Part model, mm, in its own coordinate system. Coordinates: 2 decimals unless noted, no trailing zeros. Order: outer loops, then holes, each group sorted by start corner. A loop starts at its lowest first (then second) coordinate and runs counter-clockwise, first axis right, second up.
from build123d import *

# Parameters (mm, degrees)
BOSS_EXTRUDE1_DEPTH = 0.254
SKETCH2_R           = 4.699
CUT_EXTRUDE1_DEPTH  = 1.254
SKETCH3_W           = 2.54
SKETCH3_H           = 0.635
CUT_EXTRUDE2_DEPTH  = 1.254
CUT_EXTRUDE4_DEPTH  = 1.254
CUT_EXTRUDE5_DEPTH  = 1.254


with BuildPart() as part:
    # Sketch1 → Boss-Extrude1 (new body)
    with BuildSketch(Plane.XY):
        with BuildLine():
            Line((67.21146711, 76.191723231), (8.696654013, 17.676910134))
            Line((8.696654013, 17.676910134), (7.228954972, 14.133571205))
            ThreePointArc((7.228954972, 14.133571205), (14.666587579, 6.075099489), (15.105587123, -4.88230096))
            Line((15.105587123, -4.88230096), (18.648926052, -6.35))
            Line((18.648926052, -6.35), (101.401368334, -6.35))
            ThreePointArc((101.401368334, -6.35), (93.866160503, 38.880636728), (67.21146711, 76.191723231))
        make_face()
        with BuildLine():
            Line((88.672924278, 6.35), (27.86051193, 6.35))
            ThreePointArc((27.86051193, 6.35), (26.399857642, 10.93517908), (24.190484974, 15.210228852))
            Line((24.190484974, 15.210228852), (67.191354125, 58.211098004))
            ThreePointArc((67.191354125, 58.211098004), (82.13289044, 34.020557137), (88.672924278, 6.35))
        make_face(mode=Mode.SUBTRACT)
    extrude(amount=BOSS_EXTRUDE1_DEPTH)

    # Sketch2 → Cut-Extrude1 (cut, through all)
    with BuildSketch(Plane.XY.offset(0.254)):
        with Locations((22.225, 0)):
            Circle(SKETCH2_R)
        with Locations((36.195, 0)):
            Circle(SKETCH2_R)
        with Locations((61.722, 0)):
            Circle(SKETCH2_R)
        with Locations((75.692, 0)):
            Circle(SKETCH2_R)
        with Locations((95.25, 0)):
            Circle(SKETCH2_R)
        with Locations((15.715448212, 15.715448212)):
            Circle(SKETCH2_R)
        with Locations((25.593729945, 25.593729945)):
            Circle(SKETCH2_R)
        with Locations((43.644044748, 43.644044748)):
            Circle(SKETCH2_R)
        with Locations((53.522326482, 53.522326482)):
            Circle(SKETCH2_R)
        with Locations((92.004434954, 24.652514046)):
            Circle(SKETCH2_R)
        with Locations((82.48891971, 47.625)):
            Circle(SKETCH2_R)
        with Locations((67.351920908, 67.351920908)):
            Circle(SKETCH2_R)
    extrude(amount=-CUT_EXTRUDE1_DEPTH, mode=Mode.SUBTRACT)

    # Sketch3 → Cut-Extrude2 (cut, through all)
    with BuildSketch(Plane.XY.offset(0.254)):
        Polygon((15.266435406, 24.246691527), (17.06248663, 26.042742751), (17.511499436, 25.593729945), (15.715448212, 23.797678721), align=None)
        Polygon((44.991083167, 53.971339288), (43.195031942, 52.175288063), (43.644044748, 51.726275257), (45.440095973, 53.522326482), align=None)
        with Locations((29.21, -6.0325)):
            Rectangle(SKETCH3_W, SKETCH3_H)
        with Locations((68.707, -6.0325)):
            Rectangle(SKETCH3_W, SKETCH3_H)
        Polygon((29.230733674, 38.210989795), (31.026784898, 40.007041019), (31.475797704, 39.558028213), (29.67974648, 37.761976989), align=None)
        Polygon((56.845021246, 65.825277367), (55.048970022, 64.029226143), (55.497982828, 63.580213337), (57.294034052, 65.376264561), align=None)
        with Locations((48.9585, -6.0325)):
            Rectangle(SKETCH3_W, SKETCH3_H)
        with Locations((85.471, -6.0325)):
            Rectangle(SKETCH3_W, SKETCH3_H)
        Polygon((99.935462164, 14.437711971), (100.266998693, 11.919442024), (101.526133667, 12.085210288), (101.194597138, 14.603480236), align=None)
        Polygon((93.765504959, 37.464305742), (94.938831965, 37.950313702), (93.966816047, 40.296967714), (92.793489041, 39.810959755), align=None)
        Polygon((79.327792988, 62.471156422), (80.874047017, 60.456038938), (81.88160576, 61.229165953), (80.33535173, 63.244283437), align=None)
        Polygon((13.593916116, 7.005422516), (14.565932035, 4.658768503), (15.739259041, 5.144776462), (14.767243123, 7.491430475), align=None)
    extrude(amount=-CUT_EXTRUDE2_DEPTH, mode=Mode.SUBTRACT)

    # Sketch6 → Cut-Extrude4 (cut, through all)
    with BuildSketch(Plane.XY.offset(0.254)):
        with BuildLine():
            Line((22.27103518, 28.91642471), (40.321349984, 46.966739513))
            ThreePointArc((40.321349984, 46.966739513), (46.966739513, 46.966739513), (46.966739513, 40.321349984))
            Line((46.966739513, 40.321349984), (28.91642471, 22.27103518))
            ThreePointArc((28.91642471, 22.27103518), (22.27103518, 22.27103518), (22.27103518, 28.91642471))
        make_face()
        with BuildLine():
            Line((50.199631717, 56.845021246), (64.029226143, 70.674615673))
            ThreePointArc((64.029226143, 70.674615673), (70.674615673, 70.674615673), (70.674615673, 64.029226143))
            Line((70.674615673, 64.029226143), (56.845021246, 50.199631717))
            ThreePointArc((56.845021246, 50.199631717), (50.199631717, 50.199631717), (50.199631717, 56.845021246))
        make_face()
        with BuildLine():
            Line((61.722, -4.699), (36.195, -4.699))
            ThreePointArc((36.195, -4.699), (31.496, 0), (36.195, 4.699))
            Line((36.195, 4.699), (61.722, 4.699))
            ThreePointArc((61.722, 4.699), (66.421, 0), (61.722, -4.699))
        make_face()
        with BuildLine():
            Line((95.25, -4.699), (75.692, -4.699))
            ThreePointArc((75.692, -4.699), (70.993, 0), (75.692, 4.699))
            Line((75.692, 4.699), (95.25, 4.699))
            ThreePointArc((95.25, 4.699), (99.949, 0), (95.25, -4.699))
        make_face()
        with BuildLine():
            ThreePointArc((96.543320412, 25.868704739), (92.340835395, 38.248826381), (86.558373083, 49.9745))
            ThreePointArc((86.558373083, 49.9745), (80.13941971, 51.694453372), (78.419466338, 45.2755))
            ThreePointArc((78.419466338, 45.2755), (83.658215548, 34.652367484), (87.465549496, 23.436323353))
            ThreePointArc((87.465549496, 23.436323353), (93.220625647, 20.113628588), (96.543320412, 25.868704739))
        make_face()
    extrude(amount=-CUT_EXTRUDE4_DEPTH, mode=Mode.SUBTRACT)

    # Sketch5 → Cut-Extrude5 (cut, through all)
    with BuildSketch(Plane.XY.offset(0.254)):
        Polygon((8.418953573, 4.724419036), (27.192185674, 12.500546382), (12.82377588, 26.868956175), (-0.450903843, 13.594276452), align=None)
    extrude(amount=-CUT_EXTRUDE5_DEPTH, mode=Mode.SUBTRACT)


solid = part.part
Q1. Pin check, flat tip, straight feed: pin 1 Ø5.5 at (x, y) = (22.225, 0) entering from +Z. Stop position of the tip, or through.
Results list:
pin 1: passes through
Q2. Wall check: line 1 along Y through (x, z) = (45.5, 0.2); line 2 along X through (y, z) = (57.5, 0.05); line 3 along Y through (x, z) = (39, 0.1). Give the ranges that are in metal, low to high.
Results list:
line 1: y = -6.35 to -4.7, 4.7 to 6.35, 36.52 to 38.85, 47.96 to 54.48
line 2: x = 48.52 to 50.85, 64.15 to 66.48, 67.8 to 83.76
line 3: y = -6.35 to -4.7, 4.7 to 6.35, 30.02 to 32.35, 45.65 to 47.98
Q3. Cut at C-C on z = 0.15. Count the separate pieces of the cut face and the enclosed holes in it, and give its area (3 significant figures).
Results list:
separate pieces: 1
enclosed holes: 6
area: 1,340 mm2
Q4. Cut at B-B on x = 59. Write the cut outline in (y, z).
Results list:
outline: (-6.35, 0) - (-4.7, 0) - (-4.7, 0.25) - (-6.35, 0.25) - close; (4.7, 0) - (6.35, 0) - (6.35, 0.25) - (4.7, 0.25) - close; (50.02, 0) - (52.35, 0) - (52.35, 0.25) - (50.02, 0.25) - close; (65.65, 0) - (67.98, 0) - (67.98, 0.25) - (65.65, 0.25) - close
Q5. Cut at A-A on y = 0. Write the cut outline in (x, z) (3 decimals), and give its area (3 significant figures).
Results list:
outline: (15.875, 0) - (17.526, 0) - (17.526, 0.254) - (15.875, 0.254) - close; (26.924, 0) - (31.496, 0) - (31.496, 0.254) - (26.924, 0.254) - close; (66.421, 0) - (70.993, 0) - (70.993, 0.254) - (66.421, 0.254) - close; (99.949, 0) - (101.6, 0) - (101.6, 0.254) - (99.949, 0.254) - close
area: 3.16 mm2
